Part print with two shaded views. Sizes in mm from the minimum x, y, z corner. A direction names the side the tool comes from. Round coordinates to 2 decimals unless told otherwise and drop trailing zeros. Order: outer loops, then holes, each group sorted by start corner. A loop starts at its lowest first (then second) coordinate and runs counter-clockwise, first axis right, second up. Notation, with made-up numbers: (48, 73) -> (97, 73) arc R16 ccw to (97, 92) -> close; hole circle Ø1 at (41.5, -31). An arc over 180 degrees is marked (long way). Use a Markdown table: item, result. Add a question column.
Item 1: Probe L1, parallel to X at y = 64, z = 12.5; L2, parallel to Y at x = 63, z = 15.25; L3, parallel to Y at x = 35, z = 3. List the from-to ranges inside material, lowest first.
Item 2: Slice it at B-B, the plane x = 35. Give the cut face in (y, z).
Item 3: 3-axis set-ups, long thin cutter, end or side, ignore diameter. For the marked faces 4, 5 and 6: which of +Z, -Z, +X, -X, +Y, -Y reach the whole face in a straight line?
Item 4: Two-plate mould, pull along X, no slides. Class the marked faces 1, 2 and 3: released by +X, released by -X, zero draft, split by the parting line, or undercut.
Item 5: Slice it at C-C, the plane y = 100. Give the cut face in (x, z), plus the area to 3 significant figures.
Item 6: Slice it at D-D, the plane y = 23. Give the cut face in (x, z).
Item 7: Slice it at A-A, the plane x = 78.5. Give the cut face in (y, z), plus the area to 4 significant figures.
Item 8: Pin check, flat tip, straight feed: pin 1 (15 mm diameter, centred on x = 117, y = 29.5, fed in from +Z). Stop position of the tip, or through.
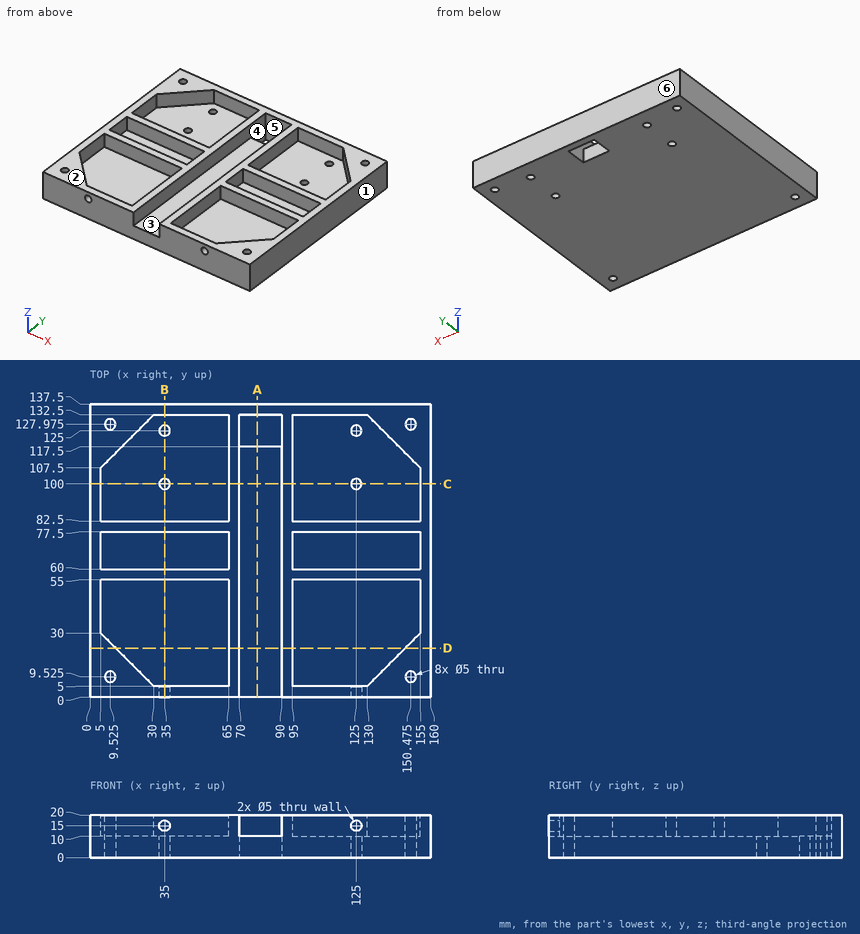
Check sheet entries:
| question | item | result |
|---|---|---|
| 1 | L1 | 0 to 5, 65 to 70, 90 to 95, 155 to 160 |
| 1 | L2 | 0 to 5, 55 to 60, 77.5 to 82.5, 132.5 to 137.5 |
| 1 | L3 | 0 to 97.5, 102.5 to 122.5, 127.5 to 137.5 |
| 2 | outline | (0, 0) -> (97.5, 0) -> (97.5, 10) -> (82.5, 10) -> (82.5, 20) -> (77.5, 20) -> (77.5, 10) -> (60, 10) -> (60, 20) -> (55, 20) -> (55, 10) -> (5, 10) -> (5, 12.5) -> (0, 12.5) -> close; (0, 17.5) -> (5, 17.5) -> (5, 20) -> (0, 20) -> close; (102.5, 0) -> (122.5, 0) -> (122.5, 10) -> (102.5, 10) -> close; (127.5, 0) -> (137.5, 0) -> (137.5, 20) -> (132.5, 20) -> (132.5, 10) -> (127.5, 10) -> close |
| 3 | face 4 | +Z |
| 3 | face 5 | +Z, -Z |
| 3 | face 6 | +Z, -Z, +X, -X, +Y |
| 4 | face 1 | released by +X |
| 4 | face 2 | zero draft |
| 4 | face 3 | undercut |
| 5 | outline | (0, 0) -> (32.5, 0) -> (32.5, 10) -> (5, 10) -> (5, 20) -> (0, 20) -> close; (37.5, 0) -> (122.5, 0) -> (122.5, 10) -> (95, 10) -> (95, 20) -> (90, 20) -> (90, 10) -> (70, 10) -> (70, 20) -> (65, 20) -> (65, 10) -> (37.5, 10) -> close; (127.5, 0) -> (160, 0) -> (160, 20) -> (155, 20) -> (155, 10) -> (127.5, 10) -> close |
| 5 | area | 1,700 mm2 |
| 6 | outline | (0, 0) -> (160, 0) -> (160, 20) -> (148, 20) -> (148, 10) -> (95, 10) -> (95, 20) -> (90, 20) -> (90, 10) -> (70, 10) -> (70, 20) -> (65, 20) -> (65, 10) -> (12, 10) -> (12, 20) -> (0, 20) -> close |
| 7 | outline | (0, 0) -> (117.5, 0) -> (117.5, 10) -> (0, 10) -> close; (132.5, 0) -> (137.5, 0) -> (137.5, 20) -> (132.5, 20) -> close |
| 7 | area | 1,275 mm2 |
| 8 | pin 1 | z = 10 |
